Here's the drawing with two shaded views (mm, measured from the low corner). I have some questions. Round coordinates to 2 decimals unless told otherwise and drop trailing zeros. Order: outer loops, then holes, each group sorted by start corner. A loop starts at its lowest first (then second) coordinate and runs counter-clockwise, first axis right, second up. Notation, with made-up numbers: (78.25, 52.25) - (89.25, 52.25) arc R16 cw to (89.25, 56.25) - close; hole circle Ø1 at (25, 83). An arc over 180 degrees is marked (long way). One line per item, written item: value.
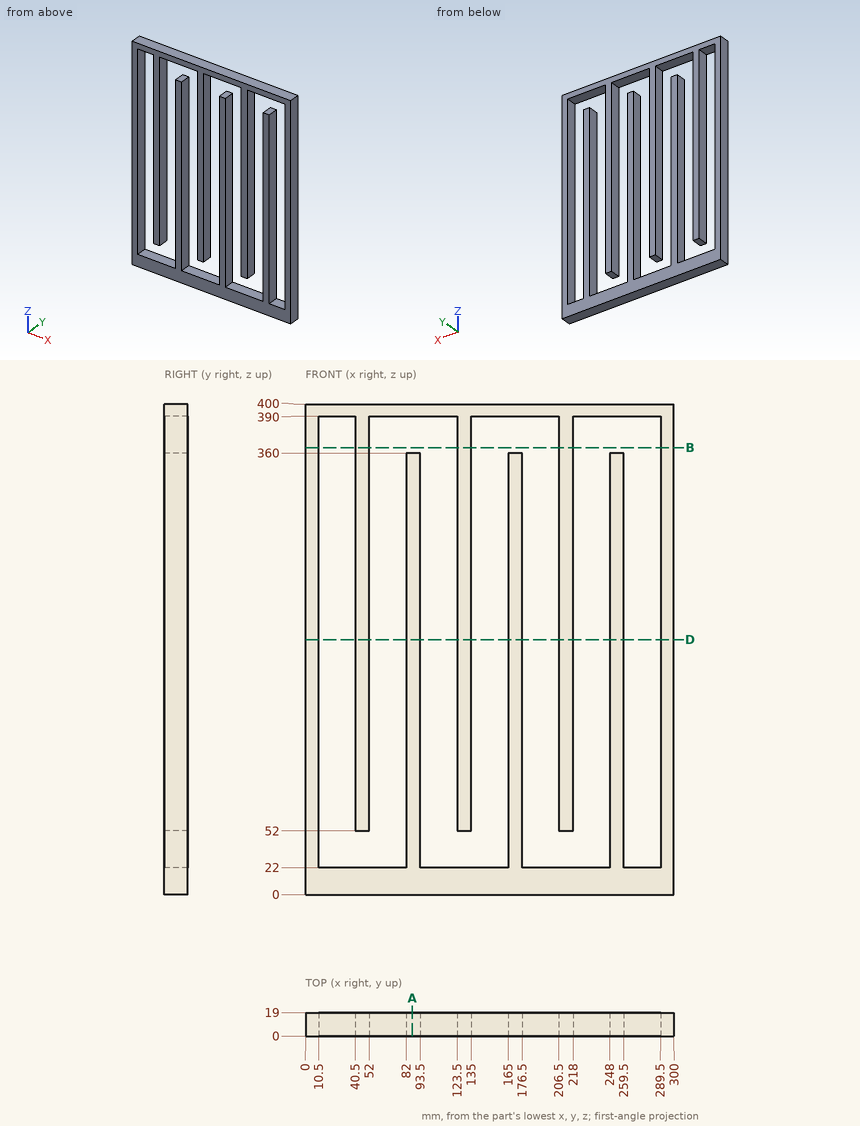
Q1. Will this pin go through, and if not, where does the flat tip stop? pin 1 (10 mm diameter, centred on x = 227, y = 13.5, fed in from -Z).
Results list:
pin 1: z = 0
Q2. If we section it at A-A, the plane x = 87: Please give me the cut outline in (y, z), then the cut area to 3 significant figures.
Results list:
outline: (0, 0) - (19, 0) - (19, 360) - (0, 360) - close; (0, 390) - (19, 390) - (19, 400) - (0, 400) - close
area: 7,030 mm²
Q3. If I drill on line 1 along X through (y, z) = (2, 376.5); line 2 along Z through (x, y) = (77, 9.5), over which ranges is the centre line in solid material (lowest first)?
Results list:
line 1: 0 to 10.5, 40.5 to 52, 123.5 to 135, 206.5 to 218, 289.5 to 300
line 2: 0 to 22, 390 to 400
Q4. If we section it at D-D, the plane z = 208: Give the number of separate pieces and of enclosed holes in the cut face, then the cut area to 3 significant figures.
Results list:
separate pieces: 8
enclosed holes: 0
area: 1,710 mm²
Q5. If we section it at B-B, the plane z = 364.5: Please give me the cut outline in (x, y), then the cut area to 3 significant figures.
Results list:
outline: (0, 0) - (10.5, 0) - (10.5, 19) - (0, 19) - close; (40.5, 0) - (52, 0) - (52, 19) - (40.5, 19) - close; (123.5, 0) - (135, 0) - (135, 19) - (123.5, 19) - close; (206.5, 0) - (218, 0) - (218, 19) - (206.5, 19) - close; (289.5, 0) - (300, 0) - (300, 19) - (289.5, 19) - close
area: 1,050 mm²
